Could you check a few things on this model? Use its own coordinates, in mm. A direction names the side the tool comes from. Give positions to 0.01 mm unless a question says otherwise; leave off trailing zeros. Write each loop counter-clockwise with the first axis right and the second up, starting at its lowest first coordinate (ties: lowest second). Pieces come first, ordered by that corner, then holes. Notation, with made-up numbers: M 73,73 L 105,73 A14 cw 105,91 Z; hole C -31.5,74 d8. An arc over 180 degrees is marked long. Use one line per item in the form item = value.
from build123d import *

# Parameters (mm, degrees)
SKETCH_R   = 2.6
SKETCH_W   = 3
SKETCH_H   = 7
SKETCH_W_2 = 20
SKETCH_H_2 = 13
PAD_DEPTH  = 5
FILLET_R   = 5


with BuildPart() as part:
    # Sketch → Pad (new body)
    with BuildSketch(Plane.XY):
        Polygon((-11.11097, 0), (11.11097, 0), (20, 40), (20, 63), (10, 108), (-10, 108), (-20, 63), (-20, 40), align=None)
        with Locations((7.5, 10)):
            Circle(SKETCH_R, mode=Mode.SUBTRACT)
        with Locations((-7.5, 10)):
            Circle(SKETCH_R, mode=Mode.SUBTRACT)
        with Locations((-6.5, 101.5)):
            Rectangle(SKETCH_W, SKETCH_H, mode=Mode.SUBTRACT)
        with Locations((6.5, 101.5)):
            Rectangle(SKETCH_W, SKETCH_H, mode=Mode.SUBTRACT)
        with Locations((0, 51.5)):
            Rectangle(SKETCH_W_2, SKETCH_H_2, mode=Mode.SUBTRACT)
        with Locations((-6.5, 69.5)):
            Rectangle(SKETCH_W, SKETCH_H, mode=Mode.SUBTRACT)
        with Locations((6.5, 69.5)):
            Rectangle(SKETCH_W, SKETCH_H, mode=Mode.SUBTRACT)
    extrude(amount=PAD_DEPTH)

    # Fillet
    fillet_edges = [part.edges().sort_by_distance(p)[0] for p in [
        (10, 108, 2.5),
        (-10, 108, 2.5),
        (20, 63, 2.5),
        (20, 40, 2.5),
        (11.11097, 0, 2.5),
        (-11.11097, 0, 2.5),
        (-20, 40, 2.5),
        (-20, 63, 2.5),
    ]]
    fillet(fillet_edges, radius=FILLET_R)


solid = part.part
1) I want a section at B-B, the plane y = 47. Please give me the cut outline in (x, z).
Checked values:
outline = M -20,0 L -10,0 L -10,5 L -20,5 Z; M 10,0 L 20,0 L 20,5 L 10,5 Z
2) If I drill on L1, parallel to Y at x = -7.5, z = 3.35; L2, parallel to Y at x = -1, z = 0.3; L3, parallel to Y at x = -8.5, z = 1.7, over which ranges is the centre line in solid material (lowest first)?
Checked values:
L1 = 0.02 to 7.4, 12.6 to 45, 58 to 66, 73 to 98, 105 to 107.77
L2 = 0 to 45, 58 to 108
L3 = 0.2 to 7.6, 12.4 to 45, 58 to 107.32
3) I want a section at D-D, the plane y = 67. Please give me the cut outline in (x, z).
Checked values:
outline = M -19.11,0 L -8,0 L -8,5 L -19.11,5 Z; M -5,0 L 5,0 L 5,5 L -5,5 Z; M 8,0 L 19.11,0 L 19.11,5 L 8,5 Z
4) For faces 1 (the flat face through (-7, 66, 2)), 2 (the flat face through (0, 43, 0)), which set-ups out of +Z, -Z, +X, -X, +Y, -Y let a thin tool reach every point of the face, with its end or its side?
Checked values:
face_1 = +Z, -Z
face_2 = -Z, +X, -X, +Y, -Y
5) Thinking about a two-plate mould opening in X: for faces 3 (the flat face through (20, 51, 2)), 4 (the flat face through (6, 98, 2)), 5 (the flat face through (0, 43, 5)), 6 (the flat face through (-8, 101, 2)), which applies, released by +X, released by -X, zero draft, split by the parting line, or undercut?
Checked values:
face_3 = released by +X
face_4 = undercut
face_5 = zero draft
face_6 = undercut
6) I want a section at A-A, the plane x = 2. Please give me the cut outline in (y, z).
Checked values:
outline = M 0,0 L 45,0 L 45,5 L 0,5 Z; M 58,0 L 108,0 L 108,5 L 58,5 Z
7) For pin 1 Ø2.5 at (y, z) = (101, 3.5) entering from -X; pin 2 Ø1.5 at (y, z) = (70, 3) entering from +X, each with a flat end and sliding along its axis, tell me the tip position at first contact or that it passes through.
Checked values:
pin_1 = -11.83
pin_2 = 18.61
8) I want a section at C-C, the plane z = 0.9. Count the separate pieces of the cut face and the enclosed holes in it, plus the area to 3 significant figures.
Checked values:
separate_pieces = 1
enclosed_holes = 7
area = 3,120 mm2
